Read the model definition and answer for the solid it produces. Units are mm, in the model's axes. Face numbers are marked on the shaded views. A direction names the side the tool comes from. Give positions to 0.01 mm unless a question says otherwise; leave off trailing zeros. Loops run counter-clockwise (first coordinate to the right, second up) from the corner with the lowest first, then second, coordinate; pieces in that order, holes last. Notation, with made-up numbers: (79.25, -30.75) - (130.25, -30.75) arc R38 ccw to (130.25, 8.25) - close; hole circle Ø4 at (58, 49). An arc over 180 degrees is marked (long way). Write item = value, one per line.
```python
from build123d import *

# Parameters (mm, degrees)
BOSS_EXTRUDE1_DEPTH = 8.5
SKETCH2_W           = 17
SKETCH2_H           = 17
CUT_EXTRUDE1_DEPTH  = 6
CUT_EXTRUDE2_DEPTH  = 3


with BuildPart() as part:
    # Sketch1 → Boss-Extrude1 (new body, symmetric)
    with BuildSketch(Plane(origin=(0, 0, 0), x_dir=(0, 0, -1), z_dir=(1, 0, 0))):
        Polygon((0, 0), (-20, 0), (-20, -3), (-11.5, -11.5), (-3, -20), (0, -20), align=None)
    extrude(amount=BOSS_EXTRUDE1_DEPTH, both=True)

    # Sketch2 → Cut-Extrude1 (cut, symmetric)
    with BuildSketch(Plane(origin=(0, 0, 0), x_dir=(0, 0, -1), z_dir=(1, 0, 0))):
        with Locations((-11.5, -11.5)):
            Rectangle(SKETCH2_W, SKETCH2_H)
    extrude(amount=CUT_EXTRUDE1_DEPTH, both=True, mode=Mode.SUBTRACT)

    # Sketch3 → Cut-Extrude2 (cut)
    with BuildSketch(Plane.XY.offset(3)):
        with BuildLine():
            Line((-3, -9), (-3, -12))
            ThreePointArc((-3, -12), (0, -15), (3, -12))
            Line((3, -12), (3, -9))
            ThreePointArc((3, -9), (0, -6), (-3, -9))
        make_face()
    cut_extrude2 = extrude(amount=-CUT_EXTRUDE2_DEPTH, mode=Mode.SUBTRACT)

    # Mirror1: Cut-Extrude2 across plane
    add(cut_extrude2.mirror(Plane(origin=(0, 0, 0), x_dir=(0, -0.707106781, 0.707106781), z_dir=(0, 0.707106781, 0.707106781))), mode=Mode.SUBTRACT)


solid = part.part
```
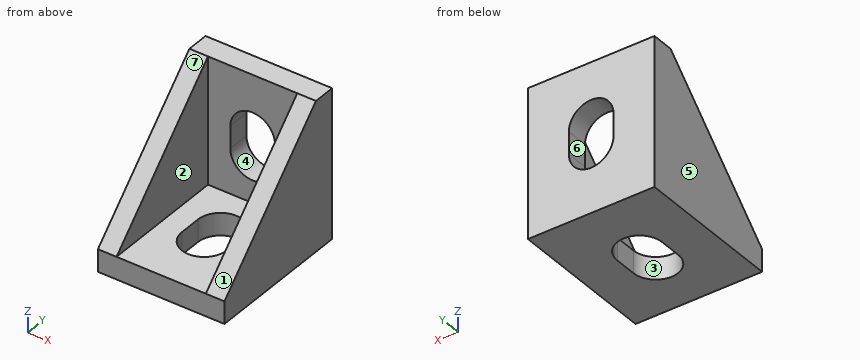
1) A cutting plane is placed at C-C on y = -7.25. Determine the outline of the cut face in (x, z), then the cut area to 3 significant figures.
Output:
outline = (-8.5, 0) - (-2.44, 0) - (-2.44, 3) - (-6, 3) - (-6, 15.75) - (-8.5, 15.75) - close; (2.44, 0) - (8.5, 0) - (8.5, 15.75) - (6, 15.75) - (6, 3) - (2.44, 3) - close
area = 100 mm²
2) A cutting plane is placed at B-B on z = 1.75. Determine the outline of the cut face in (x, y).
Output:
outline = (-8.5, -20) - (8.5, -20) - (8.5, 0) - (-8.5, 0) - close; hole (-3, -12) arc R3 ccw to (3, -12) - (3, -9) arc R3 ccw to (-3, -9) - close
3) A cutting plane is placed at D-D on z = 11. Determine the outline of the cut face in (x, y), then the cut area to 3 significant figures.
Output:
outline = (-8.5, -12) - (-6, -12) - (-6, -3) - (-3, -3) - (-3, 0) - (-8.5, 0) - close; (3, -3) - (6, -3) - (6, -12) - (8.5, -12) - (8.5, 0) - (3, 0) - close
area = 78.0 mm²
4) Each of these flat-tipped pins is pushed along its axis until it touches: P1, Ø1.5, axis at x = 5.5, y = -11, coming from the +Z side; P2, Ø6, axis at x = 6.5, z = 7.5, coming from the -Y side; P3, Ø2, axis at x = -4.5, z = 10, coming from the -Y side. Where does it stop, or does it pass through?
Output:
P1 = 12.56
P2 = -18.5
P3 = -3
5) The mould has two halves that part along X. Classify the marked faces 5, 6 and 7: pulls with the +X half, pulls with the -X half, needs draft (parallel to the pull), parting line crosses it, or undercut.
Output:
face_5 = pulls with the -X half
face_6 = undercut
face_7 = needs draft
6) A cutting plane is placed at A-A on x = 0. Determine the outline of the cut face in (y, z).
Output:
outline = (-20, 0) - (-15, 0) - (-15, 3) - (-20, 3) - close; (-6, 0) - (0, 0) - (0, 6) - (-3, 6) - (-3, 3) - (-6, 3) - close; (-3, 15) - (0, 15) - (0, 20) - (-3, 20) - close
7) Find the intervals of material crossed by probe 1 along X at (y, z) = (-5.5, 17.25); probe 2 along X at (y, z) = (-12, 1); probe 3 along Y at (x, z) = (-4.5, 18.75), in increasing order.
Output:
probe_1 = -8.5 to -6, 6 to 8.5
probe_2 = -8.5 to -3, 3 to 8.5
probe_3 = -3 to 0
8) A tool of negligible diameter and unlimited length cuts with its end or side. For the marked faces 1, 2, 3 and 4, from which of +Z, -Z, +X, -X, +Y, -Y can it reach the whole face along a straight path? Write none if from no direction.
Output:
face_1 = +Z, +X, -X, -Y
face_2 = +Z, -Y
face_3 = +Z, -Z
face_4 = +Y, -Y
